Verification items for the finished model (mm, model axes). Give positions to 0.01 mm unless a question says otherwise; leave off trailing zeros. Order: outer loops, then holes, each group sorted by start corner. A loop starts at its lowest first (then second) coordinate and runs counter-clockwise, first axis right, second up.
(1) Sectioned sample at B-B on x = 3.5. Record the cut outline in (y, z) (3 decimals).
(2) Gauge pin test, flat ends, axial feed: pin 1 (3 mm diameter, centred on x = -1.5, y = -61.5, fed in from -Z); pin 2 (1 mm diameter, centred on x = -78.5, z = 2, fed in from +Y); pin 3 (1.6 mm diameter, centred on y = -126, z = 1.5, fed in from -X) (3 decimals); pin 4 (1.6 mm diameter, centred on y = -2, z = 1, fed in from +X) (3 decimals). Record the tip position at first contact, or that the pin passes through.
(3) Sectioned sample at C-C on y = -109.5. Record the cut outline in (x, z) (3 decimals).
(4) Scan lines: L1, parallel to Y at x = -5.5, z = 0.6 (3 decimals); L2, parallel to Y at x = 70, z = 0.6; L3, parallel to X at y = -113, z = 1.75 (3 decimals). Record each from-to range of solid material in increasing order.
(5) Sectioned sample at A-A on z = 2.55. Record the cut outline in (x, y) (3 decimals).
```python
from build123d import *

# Parameters (mm, degrees)
BOSS_EXTRUDE2_DEPTH = 3.175
SKETCH2_W           = 80
SKETCH2_H           = 3.175
CUT_EXTRUDE1_DEPTH  = 4.175


with BuildPart() as part:
    # Sketch1 → Boss-Extrude2 (new body)
    with BuildSketch(Plane.XY):
        Polygon((-76.875, 0), (76.875, 0), (76.875, -15), (80.05, -15), (80.05, -85), (76.875, -85), (76.875, -124.99996875), (36.825, -124.99996875), (36.825, -128.17496875), (-36.825, -128.17496875), (-36.825, -124.99996875), (-76.825, -124.99996875), (-76.875, -85), (-80.05, -85), (-80.05, -15), (-76.875, -15), align=None)
    extrude(amount=BOSS_EXTRUDE2_DEPTH)

    # Sketch2 → Cut-Extrude1 (cut, through all)
    with BuildSketch(Plane.XY.offset(3.175)):
        with Locations((0, -1.5875)):
            Rectangle(SKETCH2_W, SKETCH2_H)
    extrude(amount=-CUT_EXTRUDE1_DEPTH, mode=Mode.SUBTRACT)


solid = part.part
```
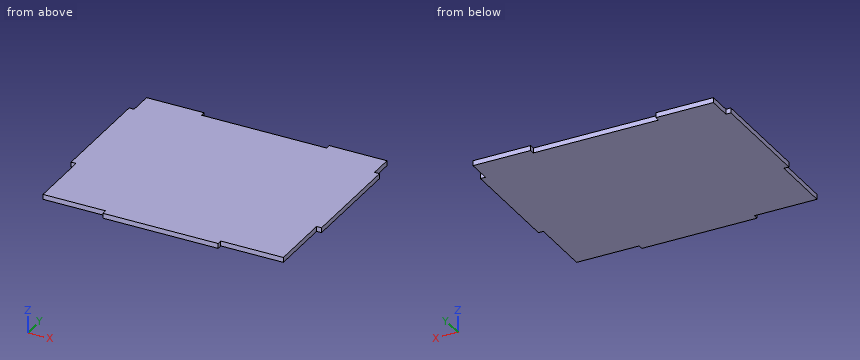
Ans:
1. outline: (-128.175, 0) - (-3.175, 0) - (-3.175, 3.175) - (-128.175, 3.175) - close
2. pin 1: stops at z = 0
2. pin 2: stops at y = -15
2. pin 3: stops at x = -36.825
2. pin 4: stops at x = 76.875
3. outline: (-76.844, 0) - (76.875, 0) - (76.875, 3.175) - (-76.844, 3.175) - close
4. L1: y = -128.175 to -3.175
4. L2: y = -125 to 0
4. L3: x = -76.84 to 76.875
5. outline: (-80.05, -85) - (-76.875, -85) - (-76.825, -125) - (-36.825, -125) - (-36.825, -128.175) - (36.825, -128.175) - (36.825, -125) - (76.875, -125) - (76.875, -85) - (80.05, -85) - (80.05, -15) - (76.875, -15) - (76.875, 0) - (40, 0) - (40, -3.175) - (-40, -3.175) - (-40, 0) - (-76.875, 0) - (-76.875, -15) - (-80.05, -15) - close
